Can you work these out from the drawing? Everything is in mm from the part's minimum corner. A direction names the side the tool comes from. Round coordinates to 2 decimals unless told otherwise and drop trailing zeros. Order: outer loops, then holes, each group sorted by start corner. A loop starts at its lowest first (then second) coordinate and runs counter-clockwise, first axis right, second up. Notation, with made-up numbers: M 38,88.25 L 46,88.25 A10 ccw 46,105.25 Z; hole C 76.25,-32 d4. An arc over 180 degrees is marked long. Use one line per item in the form item = value. Start each with the question number.
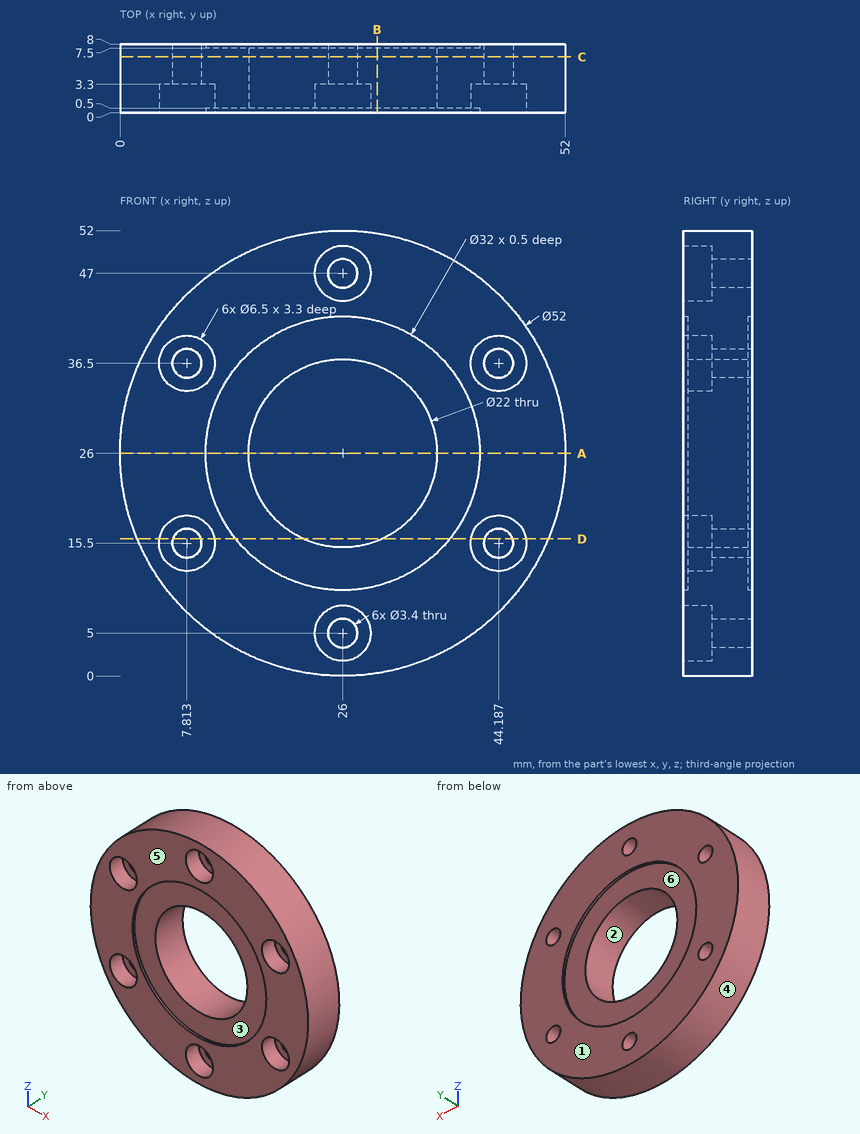
1) On a 3-axis mill with a long thin cutter (end or side, diameter ignored), from which of +Z, -Z, +X, -X, +Y, -Y can I reach the whole of each face in a straight line? I mean the marked faces 5 and 6. Say none if no direction works.
2) If we section it at C-C on y = 6.5: Write out the boundary of the cut face in (x, z).
3) If we section it at D-D on z = 16: Give the number of separate pieces and of enclosed holes in the cut face, then the cut area to 3 significant figures.
4) If I drill on line 1 (X direction, y = 0.2, z = 26); line 2 (X direction, y = 2.75, z = 35.5) (1 decimal); line 3 (Z direction, x = 8, y = 1.5) (1 decimal), over which ranges is the centre line in solid material (lowest first)?
5) If we mould it in two halves opening along Z, with no side actions, what happens to the marked faces 1, 2, 3 and 4? For each: +Z half, -Z half, draft (parallel to the pull), parting line (faces both ways), or undercut.
6) If we section it at B-B on x = 30: Write out the boundary of the cut face in (y, z), then the cut area to 3 significant figures.
7) If we section it at A-A on z = 26: Write out the boundary of the cut face in (x, y).
8) Will these pins go through, and if not, where does the flat tip stop? pin 1 Ø2 at (x, z) = (26, 5) entering from -Y (3 decimals); pin 2 Ø3 at (x, y) = (23.5, 3.5) entering from -Z; pin 3 Ø5 at (x, z) = (44, 35) entering from -Y; pin 4 Ø1 at (x, y) = (30, 1.5) entering from -Z.
Completed:
q1.face_5 = +Z, -Z, +X, -X, -Y
q1.face_6 = +Y
q2.outline = C 26,26 d52; hole C 7.81,15.5 d3.4; hole C 7.81,36.5 d3.4; hole C 26,26 d22; hole C 26,5 d3.4; hole C 26,47 d3.4; hole C 44.19,15.5 d3.4; hole C 44.19,36.5 d3.4
q3.separate_pieces = 4
q3.enclosed_holes = 0
q3.area = 222 mm²
q4.line_1 = 0 to 10, 42 to 52
q4.line_2 = 1.8 to 4.7, 10.9 to 20.5, 31.5 to 41.1, 47.3 to 50.2
q4.line_3 = 7.2 to 12.3, 18.7 to 33.3, 39.7 to 44.8
q5.face_1 = draft
q5.face_2 = undercut
q5.face_3 = undercut
q5.face_4 = parting line
q6.outline = M 0,0.31 L 8,0.31 L 8,10.51 L 7.5,10.51 L 7.5,15.75 L 0.5,15.75 L 0.5,10.51 L 0,10.51 Z; M 0,41.49 L 0.5,41.49 L 0.5,36.25 L 7.5,36.25 L 7.5,41.49 L 8,41.49 L 8,51.69 L 0,51.69 Z
q6.area = 237 mm²
q7.outline = M 0,0 L 10,0 L 10,0.5 L 15,0.5 L 15,7.5 L 10,7.5 L 10,8 L 0,8 Z; M 37,0.5 L 42,0.5 L 42,0 L 52,0 L 52,8 L 42,8 L 42,7.5 L 37,7.5 Z
q8.pin_1 = through
q8.pin_2 = 0.02
q8.pin_3 = 0
q8.pin_4 = 0.24
